The figure shows three views and two pictorial views of one solid part (mm, origin at its lowest corner). Answer the questions. Coordinates: 2 decimals unless noted, no trailing zeros. Order: outer loops, then holes, each group sorted by start corner. A loop starts at its lowest first (then second) coordinate and runs counter-clockwise, first axis right, second up. Notation, with made-up numbers: (52.25, -38.5) -> (95.25, -38.5) arc R23 ccw to (95.25, -26.5) -> close; hole circle Ø7 at (-2, -3.75). An arc over 180 degrees is marked (long way). Write item = value, one per line.
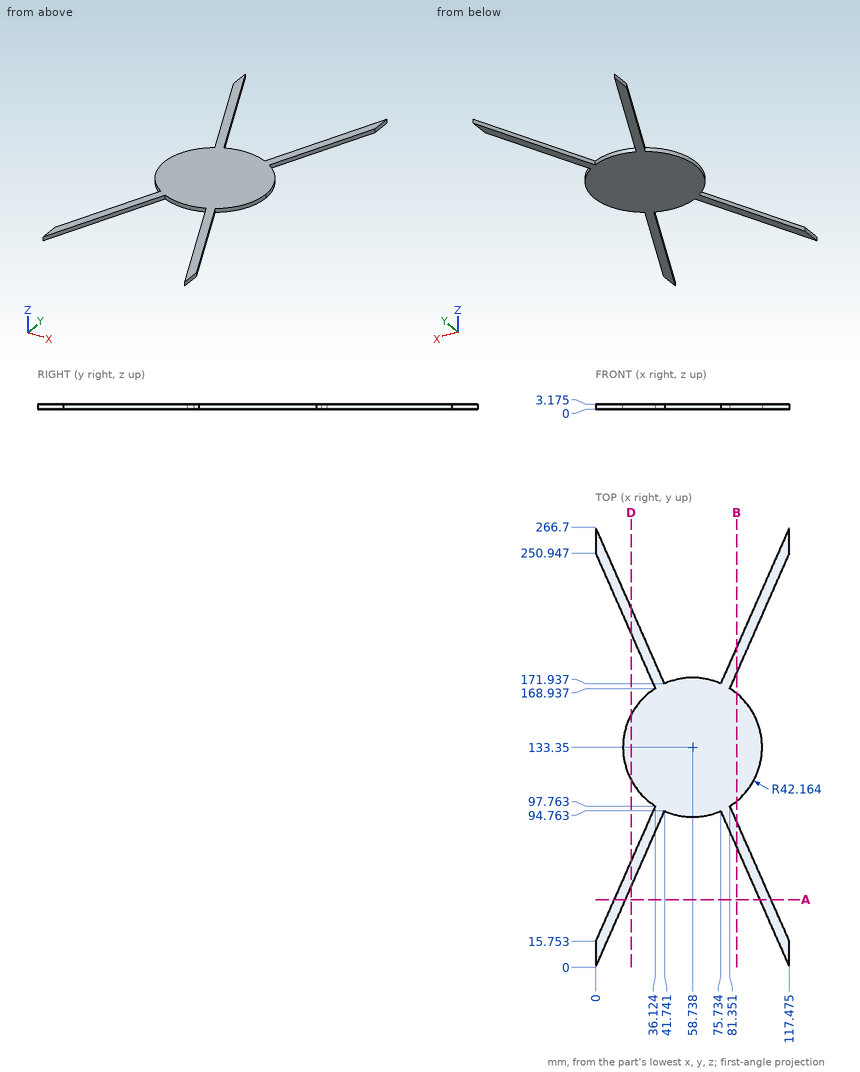
Q1. Section A-A, the plane y = 41 is taken. Give the vertices of the cut face in (x, z) (1 decimal).
The answers:
outline = (11.1, 0) -> (18.1, 0) -> (18.1, 3.2) -> (11.1, 3.2) -> close; (99.4, 0) -> (106.4, 0) -> (106.4, 3.2) -> (99.4, 3.2) -> close
Q2. Find the intervals of material crossed by line 1 along Y through (x, z) = (81.5, 2.15) (1 decimal); line 2 along Y through (x, z) = (88.5, 1.85) (1 decimal); line 3 along X through (y, z) = (44, 1.5) (1 decimal), in increasing order.
The answers:
line_1 = 81.7 to 97.4, 97.9 to 168.8, 169.3 to 185
line_2 = 65.8 to 81.5, 103.5 to 163.2, 185.2 to 200.9
line_3 = 12.4 to 19.4, 98.1 to 105
Q3. Section B-B, the plane x = 85.5 is taken. Give the vertices of the cut face in (y, z) (1 decimal).
The answers:
outline = (72.6, 0) -> (88.3, 0) -> (88.3, 3.2) -> (72.6, 3.2) -> close; (100.8, 0) -> (165.9, 0) -> (165.9, 3.2) -> (100.8, 3.2) -> close; (178.4, 0) -> (194.1, 0) -> (194.1, 3.2) -> (178.4, 3.2) -> close
Q4. This flat-tipped pin is pushed along its axis until it touches: pin 1 Ø1 at (x, z) = (46, 1) entering from +Y. Where does it stop, or does it pass through?
The answers:
pin_1 = 173.7
Q5. Section D-D, the plane x = 21.5 is taken. Give the vertices of the cut face in (y, z) (1 decimal).
The answers:
outline = (48.8, 0) -> (64.6, 0) -> (64.6, 3.2) -> (48.8, 3.2) -> close; (113.6, 0) -> (153.1, 0) -> (153.1, 3.2) -> (113.6, 3.2) -> close; (202.1, 0) -> (217.9, 0) -> (217.9, 3.2) -> (202.1, 3.2) -> close
